Design review of the part built by this model. Coordinates are the model's own, in mm. A direction names the side the tool comes from. Give positions to 0.01 mm unless a question says otherwise; leave off trailing zeros. Order: outer loops, then holes, each group sorted by start corner. A loop starts at its lowest first (then second) coordinate and runs counter-clockwise, first axis right, second up. Notation, with made-up numbers: M 1.5,39 L 33.5,39 A27 ccw 33.5,55 Z; hole C 47,28 d1. An arc over 180 degrees is marked long. Answer as a JSON object with one key per item and string values.
from build123d import *

# Parameters (mm, degrees)
CYLINDER_R              = 10
CYLINDER_DEPTH          = 60
CYLINDER001_R           = 5
CYLINDER001_DEPTH       = 10
CYLINDER002_R           = 6
CYLINDER002_DEPTH       = 38
BODY002_PLACEMENT_ANGLE = 90


with BuildPart() as part:
    # Cylinder → Cylinder (join)
    with BuildSketch(Plane(origin=(10, 0, -127), x_dir=(0, 1, 0), z_dir=(0, 0, 1))):
        Circle(CYLINDER_R)
    extrude(amount=CYLINDER_DEPTH)

    # Cone003 → Cone003 (revolve)
    with BuildSketch(Plane(origin=(10, 0, -127), x_dir=(1, 0, 0), z_dir=(0, -1, 0))):
        Polygon((0, 0), (13, 0), (0, 26), align=None)
    revolve(axis=Axis((10, 0, -127), (0, 0, 1)))

    # Cylinder001 → Cylinder001 (join)
    with BuildSketch(Plane(origin=(10, 0, -67), x_dir=(1, 0, 0), z_dir=(0, 0, 1))):
        Circle(CYLINDER001_R)
    extrude(amount=CYLINDER001_DEPTH)

    # Cylinder002 → Cylinder002 (cut)
    with BuildSketch(Plane(origin=(10, 0, -127), x_dir=(1, 0, 0), z_dir=(0, 0, 1))):
        Circle(CYLINDER002_R)
    extrude(amount=CYLINDER002_DEPTH, mode=Mode.SUBTRACT)

    # Cone → Cone (revolve, cut)
    with BuildSketch(Plane(origin=(10, 0, -89), x_dir=(1, 0, 0), z_dir=(0, -1, 0))):
        Polygon((0, 0), (6, 0), (0, 12), align=None)
    revolve(axis=Axis((10, 0, -89), (0, 0, 1)), mode=Mode.SUBTRACT)


with BuildPart() as part_1:
    # Body002 placement: moved
    add(part.part.moved(Location((10, 0, -61))).rotate(Axis((10, 0, -61), (0, 0, 1)), BODY002_PLACEMENT_ANGLE))


solid = part_1.part
(1) Insertion check: pin 1 (3 mm diameter, centred on y = 16, z = -129, fed in from +X); pin 2 (1 mm diameter, centred on x = 14, z = -171, fed in from -Y); pin 3 (10 mm diameter, centred on x = 14.5, z = -161, fed in from -Y); pin 4 (1 mm diameter, centred on y = 19.5, z = -127, fed in from -X). Each pin has a flat end and moves straight along its axis. Give the tip position at first contact, or say it passes through.
Checked values:
{"pin 1": "stops at x = 18.93", "pin 2": "stops at y = 0.63", "pin 3": "stops at y = 0", "pin 4": "passes through"}
(2) Tool access review of faces 1 (the flat face through (13, 4, -188)), 2 (the cylindrical face through (0.763, 13.83, -155.378)): name each direction out of +Z, -Z, +X, -X, +Y, -Y from which nothing blocks a thin tool from reaching the whole face with its end or side.
Checked values:
{"face 1": "-Z, +X, -X, +Y, -Y", "face 2": "+Z"}
(3) We need section B-B (z = -135). Write out the cut boundary in (x, y), plus the area to 3 significant figures.
Checked values:
{"outline": "C 10,10 d20", "area": "314 mm^2"}
(4) We need section A-A (z = -167). Write out the cut boundary in (x, y).
Checked values:
{"outline": "C 10,10 d20; hole C 10,10 d12"}
(5) To check wall thickness, follow L1, parallel to Z at x = 17.5, y = 5; L2, parallel to Y at x = 10.75, z = -171; L3, parallel to X at y = 11.5, z = -182. State the ranges of each line that lie inside material, in increasing order. Write a range as from..to.
Checked values:
{"L1": "z = -188..-128", "L2": "y = 0.03..4.05, 15.95..19.97", "L3": "x = 0.11..4.19, 15.81..19.89"}
(6) Draft analysis for pull direction Y (two halves, no side actions). For faces 3 (the cylindrical face through (13.65, 5.24, -169.27)), 4 (the flat face through (10, 10, -118)), 5 (the conical face through (11.39, 8.18, -142.58)), 6 (the cylindrical face through (8.5, 14.77, -123.07)), state which applies: +Y half, -Y half, draft (parallel to the pull), parting line (faces both ways), or undercut.
Checked values:
{"face 3": "undercut", "face 4": "draft", "face 5": "undercut", "face 6": "parting line"}
